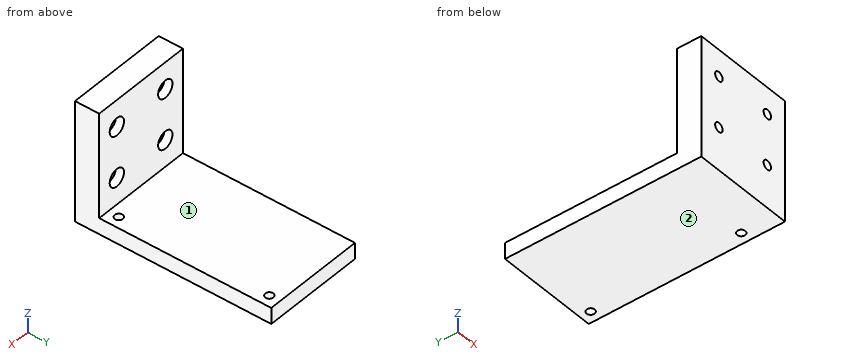
from build123d import *

# Parameters (mm, degrees)
SKETCH1_W                      = 38
SKETCH1_H                      = 45
BOSS_EXTRUDE2_DEPTH            = 9
SKETCH2_W                      = 38
SKETCH2_H                      = 6
BOSS_EXTRUDE3_DEPTH            = 64
SKETCH3_R                      = 1.5
CUT_EXTRUDE1_DEPTH             = 64
CBORE_FOR_M3_SHCS1_D           = 3.4
CBORE_FOR_M3_SHCS1_CBORE_D     = 6.5
CBORE_FOR_M3_SHCS1_CBORE_DEPTH = 3


with BuildPart() as part:
    # Sketch1 → Boss-Extrude2 (new body)
    with BuildSketch(Plane(origin=(0, 0, 0), x_dir=(1, 0, 0), z_dir=(0, 1, 0))):
        with Locations((19, 22.5)):
            Rectangle(SKETCH1_W, SKETCH1_H)
    extrude(amount=BOSS_EXTRUDE2_DEPTH)

    # Sketch2 → Boss-Extrude3 (add)
    with BuildSketch(Plane(origin=(0, 9, 0), x_dir=(1, 0, 0), z_dir=(0, 1, 0))):
        with Locations((19, 42)):
            Rectangle(SKETCH2_W, SKETCH2_H)
    extrude(amount=BOSS_EXTRUDE3_DEPTH)

    # Sketch3 → Cut-Extrude1 (cut)
    with BuildSketch(Plane.XY.offset(-39)):
        with Locations((34, 69)):
            Circle(SKETCH3_R)
        with Locations((34, 13)):
            Circle(SKETCH3_R)
    extrude(amount=-CUT_EXTRUDE1_DEPTH, mode=Mode.SUBTRACT)

    # CBORE for M3 SHCS1 (through all)
    with Locations(Plane(origin=(0, 9, 0), x_dir=(1, 0, 0), z_dir=(0, 1, 0))):
        with Locations((8, 29), (8, 10), (30, 10), (30, 29)):
            CounterBoreHole(CBORE_FOR_M3_SHCS1_D / 2, CBORE_FOR_M3_SHCS1_CBORE_D / 2, CBORE_FOR_M3_SHCS1_CBORE_DEPTH)


solid = part.part
Work out the finished part from the listing and answer in its coordinate system (mm). Face numbers are marked on the shaded views. A direction names the side the tool comes from. Give positions to 0.01 mm unless a question says otherwise; leave off trailing zeros. Loops run counter-clockwise (first coordinate to the right, second up) from the corner with the lowest first, then second, coordinate; pieces in that order, holes last. Notation, with made-up numbers: (-4.5, 70.25) - (29.5, 70.25) arc R14 ccw to (29.5, 84.25) - close; hole circle Ø6 at (-26, -2). An arc over 180 degrees is marked (long way). Answer in a Markdown table with one row per item.
(1) Section A-A (y = 69) is taken. Give the vertices of the cut face in (x, z), and give its area (3 significant figures).
Results list:
| item | result |
|---|---|
| outline | (0, -45) - (32.5, -45) - (32.5, -39) - (0, -39) - close; (35.5, -45) - (38, -45) - (38, -39) - (35.5, -39) - close |
| area | 210 mm² |
(2) Consider L1, parallel to Z at x = 8, y = 8.15; L2, parallel to Z at x = 8, y = 3.8; L3, parallel to X at y = 8, z = -29. Determine where each line is inside the solid, lowest interval first. Write a range as [from, to].
Results list:
| item | result |
|---|---|
| L1 | z = [-45, -32.25], [-25.75, -13.25], [-6.75, 0] |
| L2 | z = [-45, -30.7], [-27.3, -11.7], [-8.3, 0] |
| L3 | x = [0, 4.75], [11.25, 26.75], [33.25, 38] |
(3) Section D-D (x = 21) is taken. Give the vertices of the cut face in (y, z).
Results list:
| item | result |
|---|---|
| outline | (0, -45) - (73, -45) - (73, -39) - (9, -39) - (9, 0) - (0, 0) - close |
(4) A tool of negligible diameter and unlimited length cuts with its end or side. For the marked faces 1 and 2, from which of +Z, -Z, +X, -X, +Y, -Y can it reach the whole face along a straight path? Write none if from no direction.
Results list:
| item | result |
|---|---|
| face 1 | +Z, +X, -X, +Y |
| face 2 | -Z, +X, -X, +Y, -Y |
(5) Flat-ended cylindrical pins translate along their axes: pin 1 Ø10.5 at (x, z) = (8, -10) entering from +Y; pin 2 Ø1 at (x, y) = (26.5, 27.5) entering from +Z; pin 3 Ø5.5 at (x, z) = (8, -10) entering from +Y. Find the tip coordinate at first contact, or state that the pin passes through.
Results list:
| item | result |
|---|---|
| pin 1 | stops at y = 9 |
| pin 2 | stops at z = -39 |
| pin 3 | stops at y = 6 |
(6) Section C-C (z = -29) is taken. Give the vertices of the cut face in (x, y).
Results list:
| item | result |
|---|---|
| outline | (0, 0) - (6.3, 0) - (6.3, 6) - (4.75, 6) - (4.75, 9) - (0, 9) - close; (9.7, 0) - (28.3, 0) - (28.3, 6) - (26.75, 6) - (26.75, 9) - (11.25, 9) - (11.25, 6) - (9.7, 6) - close; (31.7, 0) - (38, 0) - (38, 9) - (33.25, 9) - (33.25, 6) - (31.7, 6) - close |
(7) Section B-B (x = 30) is taken. Give the vertices of the cut face in (y, z), and give its area (3 significant figures).
Results list:
| item | result |
|---|---|
| outline | (0, -45) - (73, -45) - (73, -39) - (9, -39) - (9, -32.25) - (6, -32.25) - (6, -30.7) - (0, -30.7) - close; (0, -27.3) - (6, -27.3) - (6, -25.75) - (9, -25.75) - (9, -13.25) - (6, -13.25) - (6, -11.7) - (0, -11.7) - close; (0, -8.3) - (6, -8.3) - (6, -6.75) - (9, -6.75) - (9, 0) - (0, 0) - close |
| area | 709 mm² |
